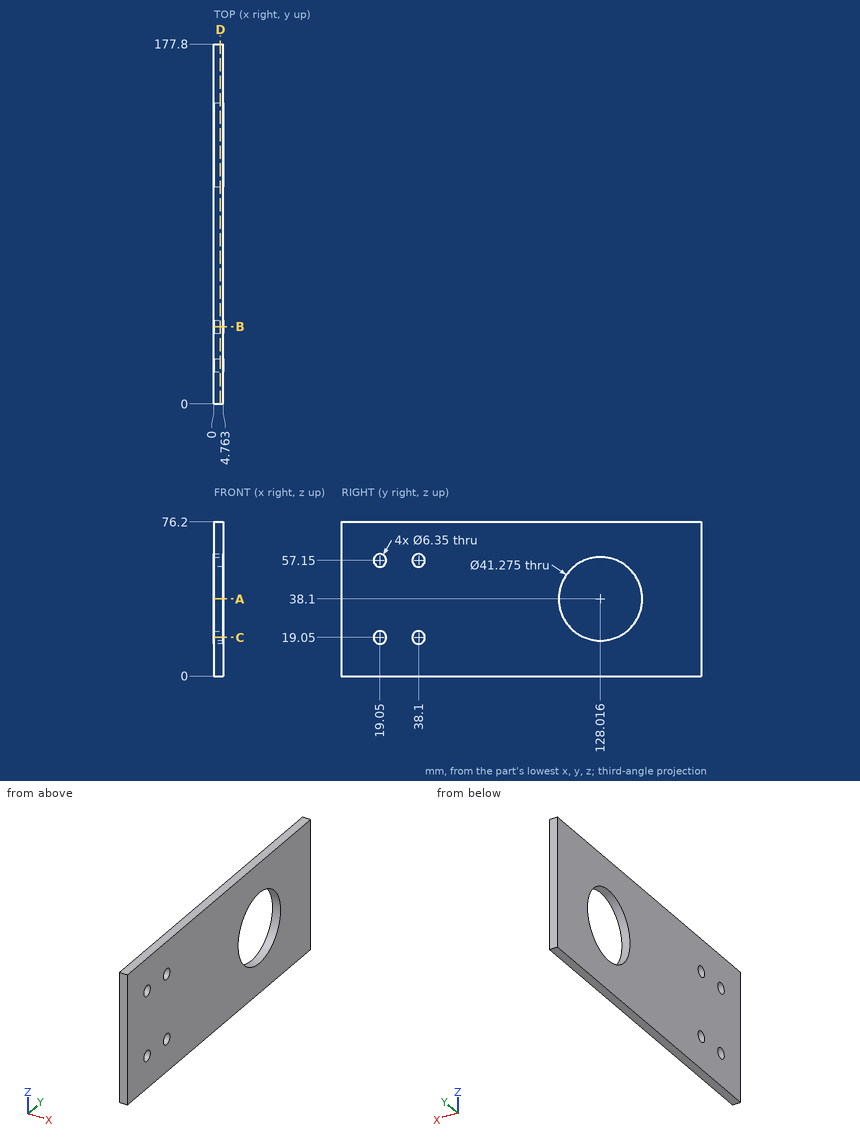
For this review, use the dimensioned drawing (mm, ordinates from the lowest corner) and the shaded views. Round coordinates to 2 decimals unless told otherwise and drop trailing zeros. Loops run counter-clockwise (first coordinate to the right, second up) from the corner with the lowest first, then second, coordinate; pieces in that order, holes last. Notation, with made-up numbers: M 1,68.5 L 46,68.5 A12 ccw 46,78.5 Z; hole C 21,-31 d4. An arc over 180 degrees is marked long. Answer as a JSON object with one key per item and string values.
(1) Take a section at B-B on y = 38.1. Give the boundary of the cut face in (x, z) (1 decimal).
Resolved:
{"outline": "M 0,0 L 4.8,0 L 4.8,15.9 L 0,15.9 Z; M 0,22.2 L 4.8,22.2 L 4.8,54 L 0,54 Z; M 0,60.3 L 4.8,60.3 L 4.8,76.2 L 0,76.2 Z"}
(2) Take a section at A-A on z = 38.1. Give the boundary of the cut face in (x, y), and give its area (3 significant figures).
Resolved:
{"outline": "M 0,0 L 4.76,0 L 4.76,107.38 L 0,107.38 Z; M 0,148.65 L 4.76,148.65 L 4.76,177.8 L 0,177.8 Z", "area": "650 mm²"}
(3) To check wall thickness, follow line 1 along Z through (x, y) = (4.2, 38.5); line 2 along Y through (x, z) = (1.8, 38.1); line 3 along Y through (x, z) = (4, 20) (1 decimal). State the ranges of each line that lie inside material, in increasing order.
Resolved:
{"line 1": "0 to 15.9, 22.2 to 54, 60.3 to 76.2", "line 2": "0 to 107.38, 148.65 to 177.8", "line 3": "0 to 16, 22.1 to 35.1, 41.1 to 118.1, 137.9 to 177.8"}
(4) Take a section at C-C on z = 19.05. Give the boundary of the cut face in (x, y) (1 decimal).
Resolved:
{"outline": "M 0,0 L 4.8,0 L 4.8,15.9 L 0,15.9 Z; M 0,22.2 L 4.8,22.2 L 4.8,34.9 L 0,34.9 Z; M 0,41.3 L 4.8,41.3 L 4.8,120.1 L 0,120.1 Z; M 0,136 L 4.8,136 L 4.8,177.8 L 0,177.8 Z"}
(5) Take a section at D-D on x = 3.2. Count the separate pieces of the cut face and the enclosed holes in it, and give its area (3 significant figures).
Resolved:
{"separate pieces": "1", "enclosed holes": "5", "area": "12,100 mm²"}
